```python
from build123d import *

# Parameters (mm, degrees)
SKETCH1_W                      = 62
SKETCH1_H                      = 108
BOSS_EXTRUDE1_DEPTH            = 6.35
M5_CLEARANCE_HOLE1_D           = 5.5
M5_CLEARANCE_HOLE1_CSINK_D     = 5.55
M5_CLEARANCE_HOLE1_CSINK_ANGLE = 100
M4_CLEARANCE_HOLE1_D           = 4.5
M4_CLEARANCE_HOLE1_CSINK_D     = 4.55
M4_CLEARANCE_HOLE1_CSINK_ANGLE = 100
CBORE_FOR_M4_SHCS1_AT_2_COUNT  = 2
CBORE_FOR_M4_SHCS1_AT_2_PITCH  = 17


with BuildPart() as part:
    # Sketch1 → Boss-Extrude1 (new body)
    with BuildSketch(Plane(origin=(0, 0, 0), x_dir=(0, 0, -1), z_dir=(1, 0, 0))):
        with Locations((31, 54)):
            Rectangle(SKETCH1_W, SKETCH1_H)
    extrude(amount=BOSS_EXTRUDE1_DEPTH)

    # M5 Clearance Hole1 (through all)
    with Locations(Plane.ZY):
        with Locations((-4, 20.5), (-4, 4.5), (-58, 4.5), (-58, 20.5)):
            CounterSinkHole(M5_CLEARANCE_HOLE1_D / 2, M5_CLEARANCE_HOLE1_CSINK_D / 2, counter_sink_angle=M5_CLEARANCE_HOLE1_CSINK_ANGLE)

    # M4 Clearance Hole1 (through all)
    with Locations(Plane(origin=(6.35, 0, 0), x_dir=(0, 0, -1), z_dir=(1, 0, 0))):
        with Locations((39.5, 82), (22.5, 82)):
            CounterSinkHole(M4_CLEARANCE_HOLE1_D / 2, M4_CLEARANCE_HOLE1_CSINK_D / 2, counter_sink_angle=M4_CLEARANCE_HOLE1_CSINK_ANGLE)

    # Sketch7 → CBORE for M4 SHCS1 (revolve, cut)
    with BuildSketch(Plane(origin=(6.35, 12, -22.5), x_dir=(0, 0, -1), z_dir=(0, 1, 0))):
        Polygon((0, 0), (0, 6.35), (2.25, 6.35), (2.25, 4), (4, 4), (4, 0.020977491), (4.025, 0), align=None)
    cbore_for_m4_shcs1 = revolve(axis=Axis((12.7, 12, -22.5), (-1, 0, 0)), mode=Mode.SUBTRACT)

    # CBORE for M4 SHCS1 at 2: CBORE for M4 SHCS1 ×2
    with Locations(*[(0, 0, -i * CBORE_FOR_M4_SHCS1_AT_2_PITCH) for i in range(1, CBORE_FOR_M4_SHCS1_AT_2_COUNT)]):
        add(cbore_for_m4_shcs1, mode=Mode.SUBTRACT)


solid = part.part
```
Can you work these out from the model? Positions are in its coordinate system, mm. A direction names the side the tool comes from. Give positions to 0.01 mm unless a question says otherwise; leave off trailing zeros. Write each loop counter-clockwise with the first axis right and the second up, starting at its lowest first coordinate (ties: lowest second). Pieces come first, ordered by that corner, then holes. Notation, with made-up numbers: (89, -30.5) - (143, -30.5) arc R32 cw to (143, -2.5) - close; hole circle Ø1 at (74.25, -36). An arc over 180 degrees is marked (long way). Write item = value, one per line. Start each with the question number.
1. Imagine slicing it at A-A (y = 82). Please give me the cut outline in (x, z) (3 decimals), and give its area (3 significant figures).
2. On a 3-axis mill with a long thin cutter (end or side, diameter ignored), from which of +Z, -Z, +X, -X, +Y, -Y can I reach the whole of each face in a straight line? I mean faces 4 (the face through (3.23, 20.621, -55.253)), 5 (the face through (2.35, 14, -38)). Say none if no direction works.
3. Thinking about a two-plate mould opening in Z: for faces 1 (the face through (3, 108, -31)), 2 (the face through (3, 53, 0)), 3 (the face through (3.23, 1.815, -3.404)), which applies, released by +Z, released by -Z, zero draft, split by the parting line, or undercut?
4. Imagine slicing it at D-D (y = 12). Please give me the cut outline in (x, z) (3 decimals), and give its area (3 significant figures).
5. For pin 1 (3.5 mm diameter, centred on y = 20.5, z = -58, fed in from -X); pin 2 (2.5 mm diameter, centred on y = 11, z = -21, fed in from +X), each with a flat end and sliding along its axis, tell me the tip position at first contact or that it passes through.
6. Please list where these lines run through material, in increasing order: line 1 (Y direction, x = 3.5, z = -4); line 2 (Z direction, x = 4, y = 82); line 3 (Y direction, x = 1.5, z = -22.5).
7. Imagine slicing it at C-C (x = 4). Count the separate pieces of the cut face and the enclosed holes in it, and give its area (3 significant figures).
8. Imagine slicing it at B-B (z = -58). Please give me the cut outline in (x, y) (3 decimals).
Worked answers:
q1.outline = (0, -62) - (6.35, -62) - (6.35, -41.775) - (6.329, -41.75) - (0, -41.75) - close; (0, -37.25) - (6.329, -37.25) - (6.35, -37.225) - (6.35, -24.775) - (6.329, -24.75) - (0, -24.75) - close; (0, -20.25) - (6.329, -20.25) - (6.35, -20.225) - (6.35, 0) - (0, 0) - close
q1.area = 337 mm2
q2.face_4 = +X, -X
q2.face_5 = +X
q3.face_1 = zero draft
q3.face_2 = released by +Z
q3.face_3 = undercut
q4.outline = (0, -62) - (6.35, -62) - (6.35, -43.525) - (6.329, -43.5) - (2.35, -43.5) - (2.35, -41.75) - (0, -41.75) - close; (0, -37.25) - (2.35, -37.25) - (2.35, -35.5) - (6.329, -35.5) - (6.35, -35.475) - (6.35, -26.525) - (6.329, -26.5) - (2.35, -26.5) - (2.35, -24.75) - (0, -24.75) - close; (0, -20.25) - (2.35, -20.25) - (2.35, -18.5) - (6.329, -18.5) - (6.35, -18.475) - (6.35, 0) - (0, 0) - close
q4.area = 309 mm2
q5.pin_1 = through
q5.pin_2 = 2.35
q6.line_1 = 0 to 1.75, 7.25 to 17.75, 23.25 to 108
q6.line_2 = -62 to -41.75, -37.25 to -24.75, -20.25 to 0
q6.line_3 = 0 to 9.75, 14.25 to 79.75, 84.25 to 108
q7.separate_pieces = 1
q7.enclosed_holes = 8
q7.area = 6,470 mm2
q8.outline = (0, 0) - (6.35, 0) - (6.35, 1.75) - (0.021, 1.75) - (0, 1.725) - close; (0, 7.275) - (0.021, 7.25) - (6.35, 7.25) - (6.35, 17.75) - (0.021, 17.75) - (0, 17.725) - close; (0, 23.275) - (0.021, 23.25) - (6.35, 23.25) - (6.35, 108) - (0, 108) - close
